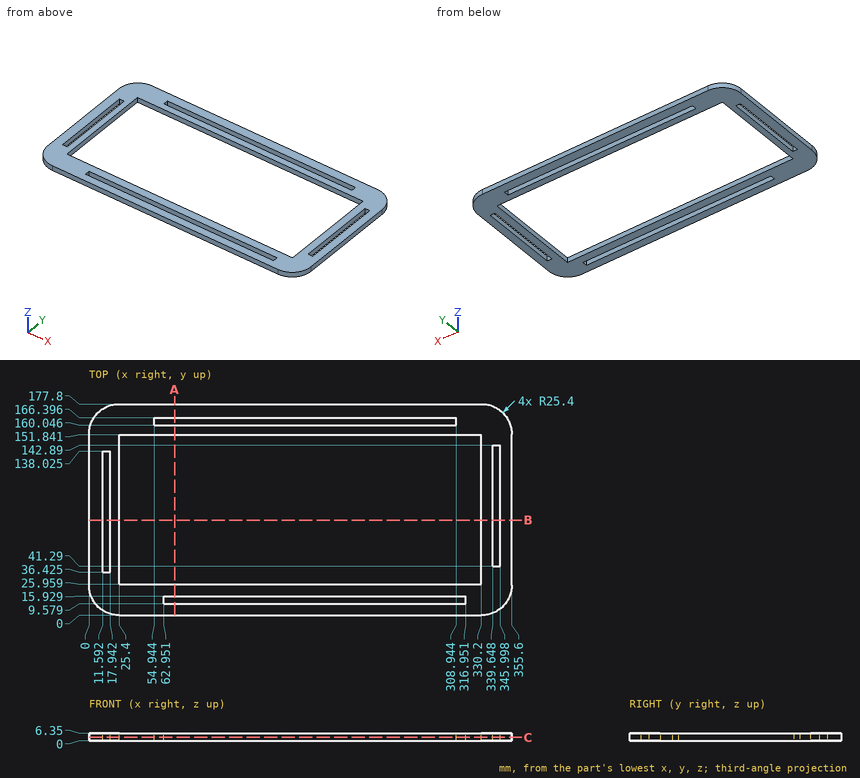
Print and shaded views of the part. All mm, measured from the part's lowest x, y and z. Give positions to 0.01 mm unless a question says otherwise; leave off trailing zeros. Write each loop counter-clockwise with the first axis right and the second up, starting at its lowest first coordinate (ties: lowest second). Pieces come first, ordered by that corner, then holes. Notation, with made-up numbers: (54.25, 58.5) - (77.25, 58.5) arc R25 cw to (77.25, 79.5) - close; hole circle Ø5 at (-11.5, -12). An arc over 180 degrees is marked (long way). One line per question, with ' | ' between items. Start each with the question number.
(1) Slice it at B-B on y = 80. Write the cut outline in (x, z), plus the area to 3 significant figures.
(2) Slice it at A-A on x = 72. Write the cut outline in (y, z), plus the area to 3 significant figures.
(3) Slice it at C-C on z = 3. Give the number of separate pieces and of enclosed holes in the cut face, plus the area to 3 significant figures.
(4) Wall check: line 1 along X through (y, z) = (121, 2.25); line 2 along Y through (x, z) = (238, 4.25); line 3 along X through (y, z) = (139, 3.5). Give the ranges that are in metal, low to high. Write a range as from..to.
(5) Pin check, flat tips, straight feed: P1, Ø1.9, axis at y = 164, z = 4.5, coming from the +X side; P2, Ø1.9, axis at x = 343.5, z = 2, coming from the -Y side (1 decimal). Stop position of each tip, or through.
Results below:
1) outline: (0, 0) - (11.59, 0) - (11.59, 6.35) - (0, 6.35) - close; (17.94, 0) - (25.4, 0) - (25.4, 6.35) - (17.94, 6.35) - close; (330.2, 0) - (339.65, 0) - (339.65, 6.35) - (330.2, 6.35) - close; (346, 0) - (355.6, 0) - (355.6, 6.35) - (346, 6.35) - close | area: 242 mm^2
2) outline: (0, 0) - (9.58, 0) - (9.58, 6.35) - (0, 6.35) - close; (15.93, 0) - (25.96, 0) - (25.96, 6.35) - (15.93, 6.35) - close; (151.84, 0) - (160.05, 0) - (160.05, 6.35) - (151.84, 6.35) - close; (166.4, 0) - (177.8, 0) - (177.8, 6.35) - (166.4, 6.35) - close | area: 249 mm^2
3) separate pieces: 1 | enclosed holes: 5 | area: 19,800 mm^2
4) line 1: 0..11.59, 17.94..25.4, 330.2..339.65, 346..355.6 | line 2: 0..9.58, 15.93..25.96, 151.84..160.05, 166.4..177.8 | line 3: 0..25.4, 330.2..339.65, 346..355.6
5) P1: x = 353.26 | P2: y = 3.2
